Geometry check sheet. Reference: the model listing, model coordinates, mm. Give positions to 0.01 mm unless a question says otherwise; leave off trailing zeros. Order: outer loops, then holes, each group sorted by start corner. A loop starts at its lowest first (then second) coordinate and runs counter-clockwise, first axis right, second up. Notation, with made-up numbers: M 75,-3 L 125,-3 A24 ccw 125,33 Z; hole C -38.75,-35.5 d11. An arc over 180 degrees is marked long. Answer as CSV lines item,"result". Start each with the question number.
Q1. Section check A-A, the plane y = -5.5. Record the boundary of the cut face in (x, z), then the cut area to 3 significant figures.
Q2. Section check B-B, the plane y = 0. Record the boundary of the cut face in (x, z).
Q3. Section check D-D, the plane z = -0.25. Record the boundary of the cut face in (x, y).
Q4. Go/stop test with a flat-tipped pin: pin 1 (1.4 mm diameter, centred on x = -5.5, y = -5.5, fed in from -Z). Record where the tip stops, or that it passes through.
Q5. Thickness scan on line 1 (Y direction, x = 5.5, z = 0.25); line 2 (X direction, y = -5.25, z = -0.75); line 3 (X direction, y = 0, z = 2.4). Record the ranges inside material, lowest first.
Q6. Mould release check, pull along Y, two halves, no side actions. Record for faces 1 (the flat face through (0, 9.5, 0)), 2 (the cylindrical face through (0.867, -3.905, -0.785)), 3 (the flat face through (9.5, 0, 0)), 4 (the flat face through (0, -9.5, 0)): +Y half, -Y half, draft (parallel to the pull), parting line (faces both ways), or undercut.
```python
from build123d import *

# Parameters (mm, degrees)
SKETCH1_W                   = 19
SKETCH1_H                   = 19
SKETCH1_R                   = 3.5
BOSS_EXTRUDE1_DEPTH         = 3.25
TAP_DRILL_FOR_M2_TAP1_D     = 1.6
TAP_DRILL_FOR_M2_TAP1_DEPTH = 11.5
SKETCH4_R                   = 4
CUT_EXTRUDE1_DEPTH          = 5


with BuildPart() as part:
    # Sketch1 → Boss-Extrude1 (new body, symmetric)
    with BuildSketch(Plane.XY):
        Rectangle(SKETCH1_W, SKETCH1_H)
        Circle(SKETCH1_R, mode=Mode.SUBTRACT)
    extrude(amount=BOSS_EXTRUDE1_DEPTH, both=True)

    # Tap Drill for M2 Tap1
    with Locations(Plane.XY.offset(3.25)):
        with Locations((-5.5, 5.5), (-5.5, -5.5), (5.5, 5.5), (5.5, -5.5)):
            Hole(TAP_DRILL_FOR_M2_TAP1_D / 2, depth=TAP_DRILL_FOR_M2_TAP1_DEPTH)

    # Sketch4 → Cut-Extrude1 (cut)
    with BuildSketch(Plane(origin=(0, 0, -3.25), x_dir=(-1, 0, 0), z_dir=(0, 0, -1))):
        Circle(SKETCH4_R)
    extrude(amount=-CUT_EXTRUDE1_DEPTH, mode=Mode.SUBTRACT)


solid = part.part
```
Answer block:
1,outline,"M -9.5,-3.25 L -6.3,-3.25 L -6.3,3.25 L -9.5,3.25 Z; M -4.7,-3.25 L 4.7,-3.25 L 4.7,3.25 L -4.7,3.25 Z; M 6.3,-3.25 L 9.5,-3.25 L 9.5,3.25 L 6.3,3.25 Z"
1,area,"103 mm2"
2,outline,"M -9.5,-3.25 L -4,-3.25 L -4,1.75 L -3.5,1.75 L -3.5,3.25 L -9.5,3.25 Z; M 3.5,1.75 L 4,1.75 L 4,-3.25 L 9.5,-3.25 L 9.5,3.25 L 3.5,3.25 Z"
3,outline,"M -9.5,-9.5 L 9.5,-9.5 L 9.5,9.5 L -9.5,9.5 Z; hole C -5.5,-5.5 d1.6; hole C -5.5,5.5 d1.6; hole C 0,0 d8; hole C 5.5,-5.5 d1.6; hole C 5.5,5.5 d1.6"
4,pin 1,"passes through"
5,line 1,"y = -9.5 to -6.3, -4.7 to 4.7, 6.3 to 9.5"
5,line 2,"x = -9.5 to -6.26, -4.74 to 4.74, 6.26 to 9.5"
5,line 3,"x = -9.5 to -3.5, 3.5 to 9.5"
6,face 1,"+Y half"
6,face 2,"undercut"
6,face 3,"draft"
6,face 4,"-Y half"
